Source: CAD feature listing. Evaluate the final solid. Frame: model axes, mm. Face numbers are marked on the shaded views. A direction names the side the tool comes from. Coordinates: 2 decimals unless noted, no trailing zeros. Loops run counter-clockwise (first coordinate to the right, second up) from the corner with the lowest first, then second, coordinate; pieces in that order, holes last.
Item 1: Section query D-D, the plane y = -78.5. Return the cut outline in (x, z), then the cut area to 3 significant figures.
Item 2: Pull-direction query (Y, two-part tool) for the marked faces 1, 2 and 3; classes: +Y half, -Y half, draft (parallel to the pull), parting line (faces both ways), or undercut.
Item 3: Line query: probe 1 along Z at (x, y) = (36.5, 5.5); probe 2 along Z at (x, y) = (-7.5, 20); probe 3 along X at (y, z) = (18, -50). Output: solid intervals per line, ascending.
Item 4: Pin query (flat end, axial travel): pin 1 Ø13 at (x, y) = (40, 40) entering from -Z; pin 2 Ø5 at (x, z) = (22, 6) entering from -Y; pin 3 Ø16 at (y, z) = (62.5, 43) entering from +X; pin 4 Ø6 at (x, y) = (40, -40) entering from -Z. Return the tip coordinate at first contact, or that it passes through.
Item 5: Section query B-B, the plane x = 0. Return the cut outline in (y, z).
Item 6: Section query A-A, the plane y = 0. Return the cut outline in (x, z).
Item 7: Section query C-C, the plane z = -42.5. Return the cut outline in (x, y).
Item 8: Reachability of the marked faces 4, 5, 6 and 7 from +Z, -Z, +X, -X, +Y, -Y: full face, straight path, thin tool, end or side. Return the list, or none.
```python
from build123d import *

# Parameters (mm, degrees)
BOSS_EXTRUDE1_DEPTH  = 10
CUT_EXTRUDE1_DEPTH   = 10
SKETCH6_W            = 20
SKETCH6_H            = 10
BOSS_EXTRUDE5_DEPTH  = 10
SKETCH7_W            = 20
SKETCH7_H            = 10
BOSS_EXTRUDE6_DEPTH  = 60
FILLET7_R            = 20
FILLET8_R            = 10
BOSS_EXTRUDE7_DEPTH  = 10
CUT_EXTRUDE7_DEPTH   = 18
FILLET7_OF_MIRROR2_R = 20
FILLET8_OF_MIRROR2_R = 10
SKETCH19_R           = 5
CUT_EXTRUDE9_DEPTH   = 30
SKETCH29_R           = 10
BOSS_EXTRUDE16_DEPTH = 15
SKETCH31_R           = 10
BOSS_EXTRUDE17_DEPTH = 15
BOSS_EXTRUDE21_DEPTH = 10
FILLET9_R            = 10
FILLET10_R           = 10
SKETCH35_R           = 10
CUT_EXTRUDE11_DEPTH  = 30
SKETCH16_R           = 25
BOSS_EXTRUDE22_DEPTH = 150


with BuildPart() as part:
    # Sketch2 → Boss-Extrude1 (new body)
    with BuildSketch(Plane.XY):
        with BuildLine():
            Line((-40, 50), (40, 50))
            ThreePointArc((40, 50), (47.071067812, 47.071067812), (50, 40))
            Line((50, 40), (50, -40))
            ThreePointArc((50, -40), (47.071067812, -47.071067812), (40, -50))
            Line((40, -50), (-40, -50))
            ThreePointArc((-40, -50), (-47.071067812, -47.071067812), (-50, -40))
            Line((-50, -40), (-50, 40))
            ThreePointArc((-50, 40), (-47.071067812, 47.071067812), (-40, 50))
        make_face()
    boss_extrude1 = extrude(amount=BOSS_EXTRUDE1_DEPTH)

    # Sketch3 → Cut-Extrude1 (cut)
    with BuildSketch(Plane.XY.offset(10)):
        with BuildLine():
            Line((-50, 40), (-50, -40))
            ThreePointArc((-50, -40), (-39.282032303, 0), (-50, 40))
        make_face()
        with BuildLine():
            Line((50, 40), (50, -40))
            ThreePointArc((50, -40), (39.282032303, 0), (50, 40))
        make_face()
    cut_extrude1 = extrude(amount=-CUT_EXTRUDE1_DEPTH, mode=Mode.SUBTRACT)

    # Sketch6 → Boss-Extrude5 (add)
    with BuildSketch(Plane.XZ.offset(50)):
        with Locations((0, 5)):
            Rectangle(SKETCH6_W, SKETCH6_H)
    boss_extrude5 = extrude(amount=BOSS_EXTRUDE5_DEPTH)

    # Sketch7 → Boss-Extrude6 (add)
    with BuildSketch(Plane.XY):
        with Locations((0, -65)):
            Rectangle(SKETCH7_W, SKETCH7_H)
    boss_extrude6 = extrude(amount=BOSS_EXTRUDE6_DEPTH)

    # Fillet7
    fillet7_edges = [part.edges().sort_by_distance(p)[0] for p in [
        (0, -70, 0),
    ]]
    fillet(fillet7_edges, radius=FILLET7_R)

    # Fillet8
    fillet8_edges = [part.edges().sort_by_distance(p)[0] for p in [
        (0, -60, 10),
    ]]
    fillet(fillet8_edges, radius=FILLET8_R)

    # Sketch8 → Boss-Extrude7 (add)
    with BuildSketch(Plane(origin=(0, -60, 0), x_dir=(1, 0, 0), z_dir=(0, 1, 0))):
        with BuildLine():
            Line((10, -60), (-10, -60))
            ThreePointArc((-10, -60), (0, -70), (10, -60))
        make_face()
    boss_extrude7 = extrude(amount=-BOSS_EXTRUDE7_DEPTH)

    # Sketch14 → Cut-Extrude7 (cut)
    with BuildSketch(Plane.XY.offset(10)):
        with BuildLine():
            Line((-39.282032303, 0), (39.282032303, 0))
            add(Edge.make_bspline(
                [(50, 40), (39.359472874, 21.350658255), (39.282032303, 0)],
                knots=[0, 0, 0, 1, 1, 1], degree=2))
            add(Edge.make_bspline(
                [(40, 50), (49.142135624, 49.142135624), (50, 40)],
                knots=[0, 0, 0, 1, 1, 1], degree=2))
            Line((40, 50), (-40, 50))
            add(Edge.make_bspline(
                [(-50, 40), (-49.142135624, 49.142135624), (-40, 50)],
                knots=[0, 0, 0, 1, 1, 1], degree=2))
            add(Edge.make_bspline(
                [(-39.282032303, 0), (-39.359472874, 21.350658255), (-50, 40)],
                knots=[0, 0, 0, 1, 1, 1], degree=2))
        make_face()
    extrude(amount=-CUT_EXTRUDE7_DEPTH, mode=Mode.SUBTRACT)


with BuildPart() as cut_extrude7_kept_piece:
    # of the separate pieces the step leaves, the one the design keeps (cut_extrude7_pieces_kept)
    add(part.part.solids().sort_by_distance((-10, -60, 20))[0])

    # Mirror2: Boss-Extrude1, Cut-Extrude1, Boss-Extrude5, Boss-Extrude6, Boss-Extrude7 across plane
    add(boss_extrude1.mirror(Plane(origin=(-39.282032303, 0, -8), x_dir=(0, 0, 1), z_dir=(0, -1, 0))))
    add(cut_extrude1.mirror(Plane(origin=(-39.282032303, 0, -8), x_dir=(0, 0, 1), z_dir=(0, -1, 0))), mode=Mode.SUBTRACT)
    add(boss_extrude5.mirror(Plane(origin=(-39.282032303, 0, -8), x_dir=(0, 0, 1), z_dir=(0, -1, 0))))
    add(boss_extrude6.mirror(Plane(origin=(-39.282032303, 0, -8), x_dir=(0, 0, 1), z_dir=(0, -1, 0))))
    add(boss_extrude7.mirror(Plane(origin=(-39.282032303, 0, -8), x_dir=(0, 0, 1), z_dir=(0, -1, 0))))

    # Fillet7 of Mirror2
    fillet7_of_mirror2_edges = [cut_extrude7_kept_piece.edges().sort_by_distance(p)[0] for p in [
        (0, 70, 0),
    ]]
    fillet(fillet7_of_mirror2_edges, radius=FILLET7_OF_MIRROR2_R)

    # Fillet8 of Mirror2
    fillet8_of_mirror2_edges = [cut_extrude7_kept_piece.edges().sort_by_distance(p)[0] for p in [
        (0, 60, 10),
    ]]
    fillet(fillet8_of_mirror2_edges, radius=FILLET8_OF_MIRROR2_R)

    # Sketch19 → Cut-Extrude9 (cut)
    with BuildSketch(Plane.XY.offset(10)):
        with Locations((-40, 40)):
            Circle(SKETCH19_R)
        with Locations((40, 40)):
            Circle(SKETCH19_R)
        with Locations((-40, -40)):
            Circle(SKETCH19_R)
        with Locations((40, -40)):
            Circle(SKETCH19_R)
    extrude(amount=-CUT_EXTRUDE9_DEPTH, mode=Mode.SUBTRACT)

    # Sketch29 → Boss-Extrude16 (add)
    with BuildSketch(Plane(origin=(0, 70, 0), x_dir=(1, 0, 0), z_dir=(0, 1, 0))):
        with Locations(Location((0, -60, 0), (0, 0, 180))):
            Circle(SKETCH29_R)
    extrude(amount=BOSS_EXTRUDE16_DEPTH)

    # Sketch30 → Revolve2 (revolve)
    with BuildSketch(Plane(origin=(0, 0, 0), x_dir=(0, 0, -1), z_dir=(1, 0, 0))):
        with BuildLine():
            Line((-60, 118.027756377), (-60, 85))
            Line((-60, 85), (-50, 85))
            ThreePointArc((-50, 85), (-42.745778116, 105.224158035), (-60, 118.027756377))
        make_face()
    revolve(axis=Axis((0, 85, 60), (0, 1, 0)))

    # Sketch31 → Boss-Extrude17 (add)
    with BuildSketch(Plane.XZ.offset(70)):
        with Locations(Location((0, 60, 0), (0, 0, 180))):
            Circle(SKETCH31_R)
    extrude(amount=BOSS_EXTRUDE17_DEPTH)

    # Sketch32 → Revolve3 (revolve)
    with BuildSketch(Plane(origin=(0, 0, 0), x_dir=(0, 0, -1), z_dir=(1, 0, 0))):
        with BuildLine():
            Line((-60, -118.027756377), (-60, -85))
            Line((-60, -85), (-70, -85))
            ThreePointArc((-70, -85), (-77.254221884, -105.224158035), (-60, -118.027756377))
        make_face()
    revolve(axis=Axis((0, -85, 60), (0, -1, 0)))

    # Sketch33 → Boss-Extrude21 (add)
    with BuildSketch(Plane.XY.offset(10)):
        with BuildLine():
            Line((-134, 10), (-39.909492971, 10))
            ThreePointArc((-39.909492971, 10), (-39.282032303, 0), (-39.909492971, -10))
            Line((-39.909492971, -10), (-134, -10))
            Line((-134, -10), (-134, 10))
        make_face()
    extrude(amount=-BOSS_EXTRUDE21_DEPTH)

    # Sketch34 → Revolve5 (revolve)
    with BuildSketch(Plane.XY):
        with BuildLine():
            Line((-178, 0), (-168.867962264, 0))
            ThreePointArc((-168.867962264, 0), (-155.201567253, 18.136805069), (-134, 10))
            Line((-134, 10), (-123.846606339, 10))
            ThreePointArc((-123.846606339, 10), (-155.08453427, 27.534478591), (-178, 0))
        make_face()
    revolve(axis=Axis((-134, 0, 0), (-1, 0, 0)))

    # Fillet9
    # the kernel refuses this fillet: 10 mm, written as the material it adds along each edge
    with BuildSketch(Plane(origin=(-150, 10, 0), x_dir=(1, 0, 0), z_dir=(0, 0, -1))) as fillet9_piece_1_section:
        with BuildLine():
            CenterArc((32.310988843, -10), FILLET9_R, 90, 58.243136141)
            ThreePointArc((23.808097042, -4.736842105), (25.09276901, -2.423886002), (26.153393661, 0))
            Line((26.153393661, 0), (32.310988843, 0))
        make_face()
    fillet9_piece_1 = revolve(axis=Axis((-150, 10, 0), (0, -1, 0)), revolution_arc=56.205276657, mode=Mode.PRIVATE)
    fillet9_piece_1 = split(fillet9_piece_1, bisect_by=Plane(origin=(-123.595029593, 11.027181376, 10), z_dir=(0, 0, -1)), keep=Keep.TOP, mode=Mode.PRIVATE)
    add(fillet9_piece_1)

    # Fillet10
    # the kernel refuses this fillet: 10 mm, written as the material it adds along each edge
    with BuildSketch(Plane(origin=(-150, -10, 0), x_dir=(0.5562190835944724, 0, 0.8310356978164808), z_dir=(-0.8310356978164808, 0, 0.5562190835944724))) as fillet10_piece_1_section:
        with BuildLine():
            CenterArc((32.310988843, -10), FILLET10_R, 90, 58.243136141)
            ThreePointArc((23.808097042, -4.736842105), (25.09276901, -2.423886002), (26.153393661, 0))
            Line((26.153393661, 0), (32.310988843, 0))
        make_face()
    fillet10_piece_1 = revolve(axis=Axis((-150, -10, 0), (0, 1, 0)), revolution_arc=56.205276657, mode=Mode.PRIVATE)
    fillet10_piece_1 = split(fillet10_piece_1, bisect_by=Plane(origin=(-123.595029593, -11.027181376, 10), z_dir=(0, 0, -1)), keep=Keep.TOP, mode=Mode.PRIVATE)
    add(fillet10_piece_1)

    # Sketch35 → Cut-Extrude11 (cut)
    with BuildSketch(Plane.XY):
        with Locations(Location((-150, 0, 0), (0, 0, 180))):
            Circle(SKETCH35_R)
    extrude(amount=CUT_EXTRUDE11_DEPTH, mode=Mode.SUBTRACT)

    # Sketch16 → Boss-Extrude22 (add)
    with BuildSketch(Plane(origin=(0, 0, 0), x_dir=(-1, 0, 0), z_dir=(0, 0, -1))):
        with Locations(Location((0, 0, 0), (0, 0, 180))):
            Circle(SKETCH16_R)
    extrude(amount=BOSS_EXTRUDE22_DEPTH)


solid = cut_extrude7_kept_piece.part
```
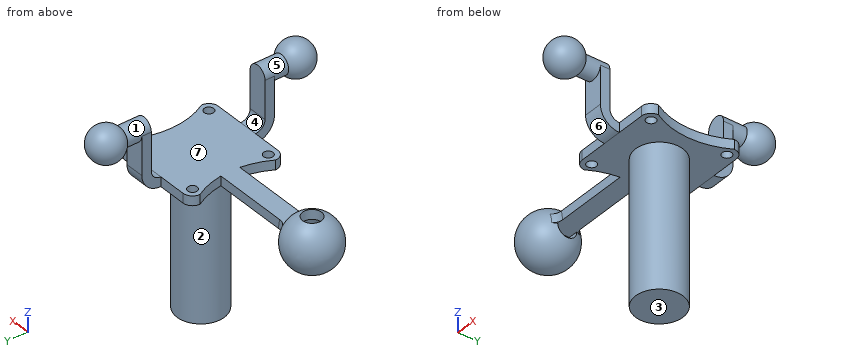
Verdict:
1. outline: circle Ø20 at (0, 60)
1. area: 314 mm2
2. face 1: undercut
2. face 2: parting line
2. face 3: draft
3. probe 1: z = 0 to 10
3. probe 2: z = -150 to 10
3. probe 3: x = -17.35 to 17.35
4. pin 1: stops at z = 0
4. pin 2: stops at y = -50
4. pin 3: stops at x = 10
4. pin 4: passes through
5. outline: (-85, 50) - (-70, 50) - (-70, 20) arc R20 ccw to (-50, 0) - (-25, 0) - (-25, -150) - (25, -150) - (25, 0) - (50, 0) arc R20 ccw to (70, 20) - (70, 50) - (85, 50) arc R18.03 ccw (long way) to (85, 70) - (60, 70) - (60, 20) arc R10 cw to (50, 10) - (-50, 10) arc R10 cw to (-60, 20) - (-60, 70) - (-85, 70) arc R18.03 ccw (long way) to start
6. outline: (-160, 16) - (-160, 26.15) arc R28 ccw (long way) to (-123.85, -10) - (-134, -10) arc R18.87 cw (long way) to start; (-140, 16) arc R18.87 cw to (-134, 10) - (-134, 0) - (-25, 0) - (-25, -150) - (25, -150) - (25, 0) - (39.28, 0) - (39.28, 10) - (-123.85, 10) arc R28 ccw to (-140, 26.15) - close
7. outline: circle Ø50 at (0, 0)
8. face 4: +Z, +X, -X
8. face 5: none
8. face 6: -Z, +X, -X, -Y
8. face 7: +Z, +X
